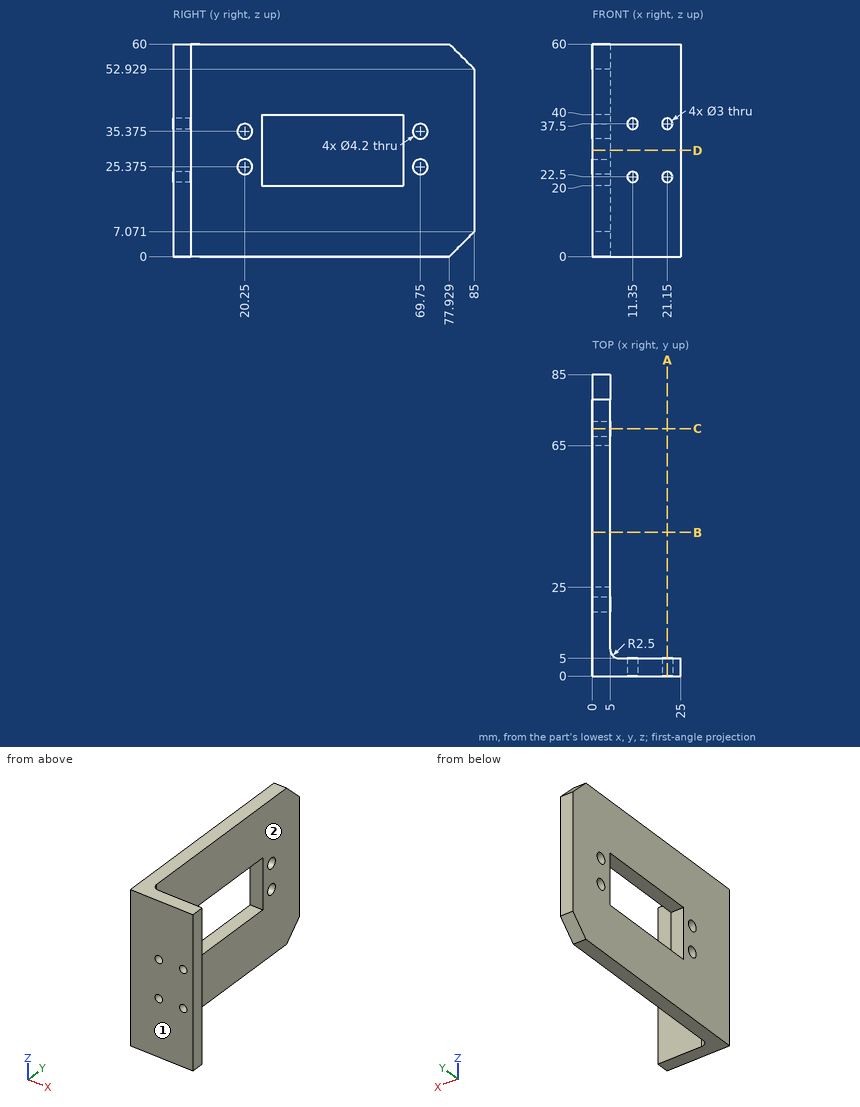
Study the drawing (mm; zero at the part's minimum x, y, z) and answer. A direction names the side the tool comes from. Round coordinates to 2 decimals unless told otherwise and drop trailing zeros. Write each loop counter-clockwise with the first axis right and the second up, starting at its lowest first coordinate (ties: lowest second). Pieces come first, ordered by that corner, then holes.
Q1. Find section A-A on x = 21.15. Determine the outline of the cut face in (y, z), and give its area (3 significant figures).
Values:
outline: (0, 0) - (5, 0) - (5, 21) - (0, 21) - close; (0, 24) - (5, 24) - (5, 36) - (0, 36) - close; (0, 39) - (5, 39) - (5, 60) - (0, 60) - close
area: 270 mm2
Q2. Find section D-D on z = 30. Determine the outline of the cut face in (x, y).
Values:
outline: (0, 0) - (25, 0) - (25, 5) - (7.5, 5) arc R2.5 cw to (5, 7.5) - (5, 25) - (0, 25) - close; (0, 65) - (5, 65) - (5, 85) - (0, 85) - close
Q3. Straight lines are drawn through the part: line 1 (Z direction, x = 21.15, y = 3.35); line 2 (Y direction, x = 2.5, z = 31); line 3 (Z direction, x = 3, y = 51.5). For each, find the intervals that lie inside material, in ascending order.
Values:
line 1: z = 0 to 21, 24 to 36, 39 to 60
line 2: y = 0 to 25, 65 to 85
line 3: z = 0 to 20, 40 to 60
Q4. Flat-ended cylindrical pins translate along their axes: P1, Ø5.5, axis at y = 69.75, z = 35.37, coming from the +X side; P2, Ø10, axis at x = 14.5, z = 45, coming from the +Y side. Find the tip coordinate at first contact, or state that the pin passes through.
Values:
P1: stops at x = 5
P2: stops at y = 5
Q5. Find section C-C on y = 69.75. Determine the outline of the cut face in (x, z) (1 decimal).
Values:
outline: (0, 0) - (5, 0) - (5, 23.3) - (0, 23.3) - close; (0, 27.5) - (5, 27.5) - (5, 33.3) - (0, 33.3) - close; (0, 37.5) - (5, 37.5) - (5, 60) - (0, 60) - close
Q6. A tool of negligible diameter and unlimited length cuts with its end or side. For the marked faces 1 and 2, from which of +Z, -Z, +X, -X, +Y, -Y can it reach the whole face along a straight path? Write none if from no direction.
Values:
face 1: +Z, -Z, +X, -X, -Y
face 2: +Z, -Z, +X, +Y
Q7. Find section B-B on y = 40.5. Determine the outline of the cut face in (x, z).
Values:
outline: (0, 0) - (5, 0) - (5, 20) - (0, 20) - close; (0, 40) - (5, 40) - (5, 60) - (0, 60) - close
